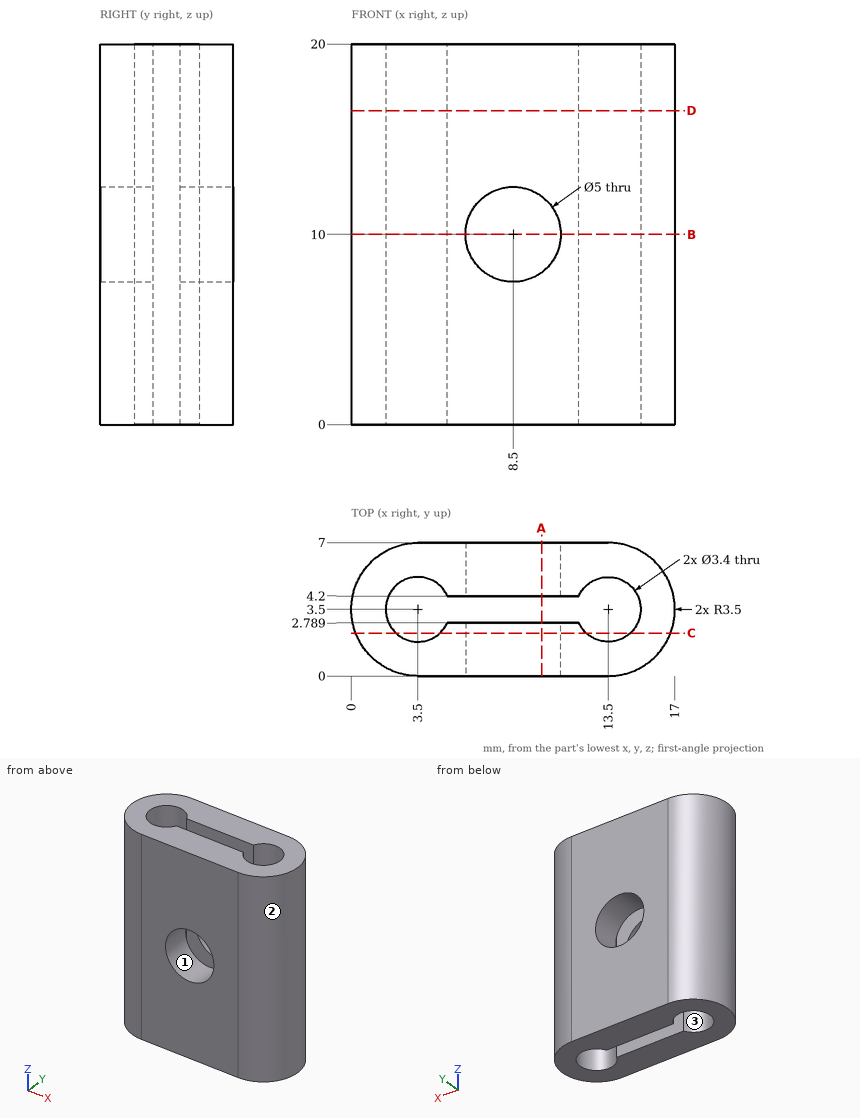
Print and shaded views of the part. All mm, measured from the part's lowest x, y and z. Coordinates: 2 decimals unless noted, no trailing zeros. Loops run counter-clockwise (first coordinate to the right, second up) from the corner with the lowest first, then second, coordinate; pieces in that order, holes last. Notation, with made-up numbers: (-38, -15) -> (18, -15) arc R22 cw to (18, 10) -> close; hole circle Ø4 at (30, 40). An arc over 180 degrees is marked (long way). Use one line per item in the form item = value. Start each with the question number.
(1) Probe probe 1 along X at (y, z) = (3.5, 15.25); probe 2 along Y at (x, z) = (3.5, 9.5); probe 3 along Z at (x, y) = (8.5, 6.45). List the from-to ranges inside material, lowest first. Write a range as from..to.
(2) Cut at A-A on x = 10. Give the cut face in (y, z).
(3) Pull direction Y, two halves, no side cores. Call the marked faces 1, 2 and 3: pulls with the +Y half, pulls with the -Y half, needs draft (parallel to the pull), parting line crosses it, or undercut.
(4) Cut at D-D on z = 16.5. Give the cut face in (x, y), and give its area (3 significant figures).
(5) Flat gauge pins, fed straight in: pin 1 (1.5 mm diameter, centred on y = 2.5, z = 15, fed in from -X); pin 2 (1 mm diameter, centred on x = 2, z = 6.5, fed in from -Y); pin 3 (3 mm diameter, centred on x = 8.5, z = 10, fed in from -Y). Where does each tip first touch, or does it go through?
(6) Cut at C-C on y = 2.25. Give the cut face in (x, z), and give its area (3 significant figures).
(7) Cut at B-B on z = 10. Give the cut face in (x, y), and give its area (3 significant figures).
Values:
q1.probe_1 = 0..1.8, 15.2..17
q1.probe_2 = 0..1.8, 5.2..7
q1.probe_3 = 0..7.5, 12.5..20
q2.outline = (0, 0) -> (2.79, 0) -> (2.79, 8) -> (0, 8) -> close; (0, 12) -> (2.79, 12) -> (2.79, 20) -> (0, 20) -> close; (4.2, 0) -> (7, 0) -> (7, 8) -> (4.2, 8) -> close; (4.2, 12) -> (7, 12) -> (7, 20) -> (4.2, 20) -> close
q3.face_1 = needs draft
q3.face_2 = parting line crosses it
q3.face_3 = undercut
q4.outline = (3.5, 0) -> (13.5, 0) arc R3.5 ccw to (13.5, 7) -> (3.5, 7) arc R3.5 ccw to start; hole (5.04, 2.79) -> (11.96, 2.79) arc R1.7 ccw (long way) to (11.95, 4.2) -> (5.05, 4.2) arc R1.7 ccw (long way) to start
q4.area = 80.9 mm2
q5.pin_1 = 0.01
q5.pin_2 = 0.15
q5.pin_3 = through
q6.outline = (0.23, 0) -> (2.35, 0) -> (2.35, 20) -> (0.23, 20) -> close; (4.65, 0) -> (12.35, 0) -> (12.35, 20) -> (4.65, 20) -> close; (14.65, 0) -> (16.77, 0) -> (16.77, 20) -> (14.65, 20) -> close; hole circle Ø5 at (8.5, 10)
q6.area = 219 mm2
q7.outline = (3.5, 0) -> (6, 0) -> (6, 2.79) -> (5.04, 2.79) arc R1.7 cw (long way) to (5.05, 4.2) -> (6, 4.2) -> (6, 7) -> (3.5, 7) arc R3.5 ccw to start; (11, 0) -> (13.5, 0) arc R3.5 ccw to (13.5, 7) -> (11, 7) -> (11, 4.2) -> (11.95, 4.2) arc R1.7 cw (long way) to (11.96, 2.79) -> (11, 2.79) -> close
q7.area = 52.9 mm2
